Build history of the part. All positions in model axes, mm. Face numbers are marked on the shaded views. Round coordinates to 2 decimals unless told otherwise and drop trailing zeros. Write each loop counter-clockwise with the first axis right and the second up, starting at its lowest first coordinate (ties: lowest second). Pieces come first, ordered by that corner, then holes. Notation, with made-up numbers: (4, 83) - (53, 83) arc R10 ccw to (53, 90) - close; hole circle Ø8 at (47, 7.25). An arc over 180 degrees is marked (long way). Write each question's results on one line, items separated by ' | '.
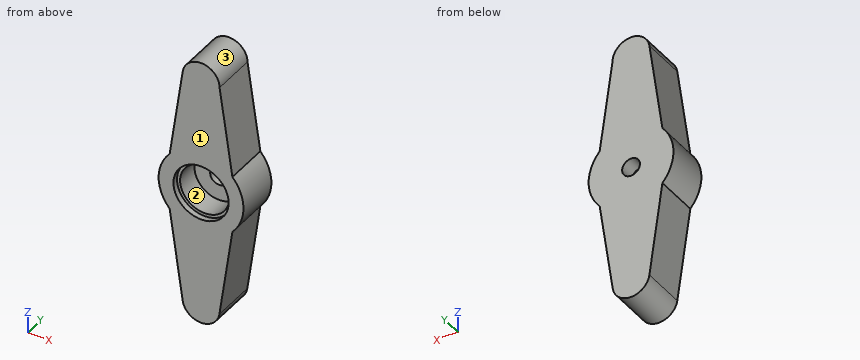
Autodesk Inventor part; units mm, degrees
ref_plane "YZ Plane" through (0, 0, 0) normal (1, 0, 0) x (0, 1, 0)
ref_plane "XZ Plane" through (0, 0, 0) normal (0, 1, 0) x (-1, 0, 0)
ref_plane "XY Plane" through (0, 0, 0) normal (0, 0, 1) x (1, 0, 0)
sketch "Sketch1" plane through (0, 0, 0) normal (0, 1, 0) x (-1, 0, 0)
  circle A0 centre (0, 0) radius 5.95
  circle A1 centre (0, -16.35) radius 2.6
  line L0 (4.4, -4.0053) -> (2.5736, -16.7197)
  circle A2 centre (0, 16.35) radius 2.6
  line L1 (4.4, 4.0053) -> (2.5736, 16.7197)
  line L2 (-4.4, 4.0053) -> (-2.6, 16.35)
  line L3 (-4.4, -4.0053) -> (-2.5736, -16.7197)
  dimension "d0" = 11.9
  dimension "d1" = 5.2
  dimension "d2" = 4.4
  dimension "d3" = 5.2
  dimension "d4" = 16.35
  dimension "d5" = 16.35
  dimension "d6" = 4.4
  dimension "d7" = 4.4
  dimension "d8" = 4.4
  dimension "d9" = 0
extrude "Extrusion1" add sketch "Sketch1" along normal blind 2.2
sketch "Sketch2" plane through (0, 0, 0) normal (0, -1, 0) x (1, 0, 0)
  circle A0 centre (0, 0) radius 3.8734
  circle A1 centre (0, 0) radius 3.45
  dimension "d12" = 6.9
extrude "Extrusion2" add sketch "Sketch2" along normal blind 3.2
sketch "Sketch3" plane through (0, 2.2, 0) normal (0, 1, 0) x (1, 0, 0)
  circle A0 centre (0, 0) radius 1.25
  dimension "d15" = 2.5
extrude "Extrusion3" cut sketch "Sketch3" against normal blind 2.2
thicken "Thicken2" operation add thickness 4 both sides no extend neighbours no toward (0, -1, 0) faces at (0.1556, 0, -12.4282)
properties part number "servo_attach"
(1) Flat gauge pins, fed straight in: pin 1 Ø3.5 at (x, z) = (-0.5, 0) entering from -Y; pin 2 Ø3 at (x, y) = (3.5, -2) entering from +Z; pin 3 Ø6 at (x, z) = (0.5, -3.5) entering from -Y; pin 4 Ø3 at (y, z) = (-3.5, -10.5) entering from -X. Where does each tip first touch, or does it go through?
Worked answers:
pin 1: stops at y = 0 | pin 2: stops at z = 18.01 | pin 3: stops at y = -4 | pin 4: stops at x = -3.68
(2) Slice it at B-B, the plane x = 0. Write the cut outline in (y, z), and give its area (3 significant figures).
Worked answers:
outline: (-4, -18.95) - (2.2, -18.95) - (2.2, -1.25) - (0, -1.25) - (0, -3.45) - (-3.2, -3.45) - (-3.2, -3.87) - (-4, -3.87) - close; (-4, 3.87) - (-3.2, 3.87) - (-3.2, 3.45) - (0, 3.45) - (0, 1.25) - (2.2, 1.25) - (2.2, 18.95) - (-4, 18.95) - close | area: 201 mm2
(3) Two-plate mould, pull along X, no slides. Class the marked faces 1, 2 and 3: released by +X, released by -X, zero draft, split by the parting line, or undercut.
Worked answers:
face 1: zero draft | face 2: undercut | face 3: split by the parting line
(4) Drill centre lines: probe 1 along X at (y, z) = (1.5, 0); probe 2 along Y at (x, z) = (1, 2.5); probe 3 along Z at (x, y) = (4.5, -3). Where is each one in solid material? Low to high. Write a range as [from, to].
Worked answers:
probe 1: x = [-5.95, -1.25], [1.25, 5.95] | probe 2: y = [0, 2.2] | probe 3: z = [-3.89, 3.89]
(5) Slice it at A-A, the plane z = 0. Write the cut outline in (x, y), and give its area (3 significant figures).
Worked answers:
outline: (-5.95, -4) - (-3.87, -4) - (-3.87, -3.2) - (-3.45, -3.2) - (-3.45, 0) - (-1.25, 0) - (-1.25, 2.2) - (-5.95, 2.2) - close; (1.25, 0) - (3.45, 0) - (3.45, -3.2) - (3.87, -3.2) - (3.87, -4) - (5.95, -4) - (5.95, 2.2) - (1.25, 2.2) - close | area: 40.0 mm2
(6) Slice it at C-C, the plane y = -1. Write the cut outline in (x, z), and give its area (3 significant figures).
Worked answers:
outline: (-4.4, -4.01) - (-2.57, -16.72) arc R2.6 ccw to (2.57, -16.72) - (4.4, -4.01) arc R5.95 ccw to (4.4, 4.01) - (2.6, 16.35) arc R2.6 ccw to (-2.57, 16.72) - (-4.4, 4.01) arc R5.95 ccw to start; hole circle Ø6.9 at (0, 0) | area: 245 mm2
(7) Slice it at D-D, the plane x = 1.75. Write the cut outline in (y, z), and give its area (3 significant figures).
Worked answers:
outline: (-4, -18.27) - (2.2, -18.27) - (2.2, 18.27) - (-4, 18.27) - (-4, 3.46) - (-3.2, 3.46) - (-3.2, 2.97) - (0, 2.97) - (0, -2.97) - (-3.2, -2.97) - (-3.2, -3.46) - (-4, -3.46) - close | area: 202 mm2
